Work out the finished part from the listing and answer in its coordinate system (mm). Face numbers are marked on the shaded views. Round coordinates to 2 decimals unless told otherwise and drop trailing zeros. Order: outer loops, then holes, each group sorted by start corner. A loop starts at its lowest first (then second) coordinate and runs counter-clockwise, first axis right, second up. Notation, with made-up numbers: (36, 84.5) -> (47, 84.5) arc R25 cw to (47, 102.5) -> close; hole circle Ø2 at (28, 47). An arc over 180 degrees is marked (long way). Use one line per item in the form item = value.
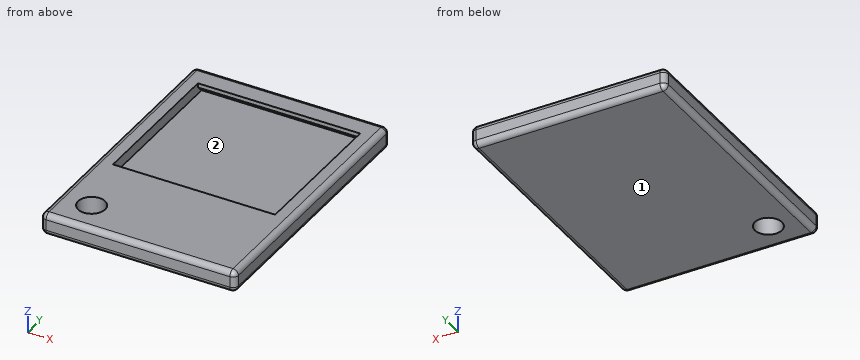
```python
from build123d import *

# Parameters (mm, degrees)
F0_W          = 36
F0_H          = 50
F1_DEPTH      = 4
F2_W          = 30
F2_H          = 30
F3_DEPTH      = 2
F4_R          = 1
F6_DEPTH      = 15
F6_DEPTH_BACK = 15
F8_DEPTH      = 15
F8_DEPTH_BACK = 15
F9_R          = 2.5
F10_DEPTH     = 4.001


with BuildPart() as f1:
    # F0 (on Top) → F1 (new body)
    with BuildSketch(Plane.XY):
        Rectangle(F0_W, F0_H)
    extrude(amount=F1_DEPTH)

    # F2 (on face) → F3 (cut)
    with BuildSketch(Plane.XY.offset(4)):
        with Locations((0, 7)):
            Rectangle(F2_W, F2_H)
    extrude(amount=-F3_DEPTH, mode=Mode.SUBTRACT)

    # F4
    f4_edges = [f1.edges().sort_by_distance(p)[0] for p in [
        (0, -25, 4),
        (18, 0, 4),
        (0, 25, 4),
        (-18, 0, 4),
        (18, -25, 2),
        (-18, -25, 2),
        (18, 25, 2),
        (18, 0, 0),
        (0, -25, 0),
        (-18, 0, 0),
        (0, 25, 0),
        (-18, 25, 2),
    ]]
    fillet(f4_edges, radius=F4_R)

    # F5 (on Right) → F6 (join, two sides)
    with BuildSketch(Plane.YZ) as f6_sk:
        Polygon((-6.8, 4), (-8, 4), (-8, 2), (-6.8, 3.2), align=None)
    extrude(amount=F6_DEPTH)
    extrude(f6_sk.sketch, amount=-F6_DEPTH_BACK)

    # F7 (on Right) → F8 (join, two sides)
    with BuildSketch(Plane.YZ) as f8_sk:
        Polygon((22, 2), (22, 4), (20.8, 4), (20.8, 3.2), align=None)
    extrude(amount=F8_DEPTH)
    extrude(f8_sk.sketch, amount=-F8_DEPTH_BACK)

    # F9 (on face) → F10 (cut, through all)
    with BuildSketch(Plane.XY.offset(4)):
        with Locations((-12, -19)):
            Circle(F9_R)
    extrude(amount=-F10_DEPTH, mode=Mode.SUBTRACT)


solid = f1.part
```
Item 1: The part is cut by section A-A, the plane y = -19. Give the vertices of the cut face in (x, z), and give its area (3 significant figures).
Findings:
outline = (-18, 1) arc R1 ccw to (-17, 0) -> (-14.5, 0) -> (-14.5, 4) -> (-17, 4) arc R1 ccw to (-18, 3) -> close; (-9.5, 0) -> (17, 0) arc R1 ccw to (18, 1) -> (18, 3) arc R1 ccw to (17, 4) -> (-9.5, 4) -> close
area = 123 mm^2
Item 2: Flat-ended cylindrical pins translate along their axes: P1, Ø10, axis at x = 4.5, y = 9.5, coming from the +Z side; P2, Ø0.6, axis at x = -6, z = 3.5, coming from the -Y side; P3, Ø4.5, axis at x = -12, y = -19, coming from the +Z side. Find the tip coordinate at first contact, or state that the pin passes through.
Findings:
P1 = 2
P2 = -24.98
P3 = through
Item 3: Consider line 1 along Y through (x, z) = (-12, 1.9); line 2 along Y through (x, z) = (-12, 2.9); line 3 along X through (y, z) = (-6, 2.35). Determine where each line is inside the solid, lowest interval first.
Findings:
line_1 = -25 to -21.5, -16.5 to 25
line_2 = -25 to -21.5, -16.5 to -7.1, 21.1 to 25
line_3 = -18 to -15, 15 to 18
Item 4: The part is cut by section B-B, the plane x = -13.5. Give the vertices of the cut face in (y, z).
Findings:
outline = (-25, 1) arc R1 ccw to (-24, 0) -> (-21, 0) -> (-21, 4) -> (-24, 4) arc R1 ccw to (-25, 3) -> close; (-17, 0) -> (24, 0) arc R1 ccw to (25, 1) -> (25, 3) arc R1 ccw to (24, 4) -> (20.8, 4) -> (20.8, 3.2) -> (22, 2) -> (-8, 2) -> (-6.8, 3.2) -> (-6.8, 4) -> (-17, 4) -> close
Item 5: Determine the mould class of the marked faces 1 and 2 for opening direction X: released by +X, released by -X, zero draft, split by the parting line, or undercut.
Findings:
face_1 = zero draft
face_2 = undercut
Item 6: The part is cut by section C-C, the plane y = 16. Give the vertices of the cut face in (x, z), and give its area (3 significant figures).
Findings:
outline = (-18, 1) arc R1 ccw to (-17, 0) -> (17, 0) arc R1 ccw to (18, 1) -> (18, 3) arc R1 ccw to (17, 4) -> (15, 4) -> (15, 2) -> (-15, 2) -> (-15, 4) -> (-17, 4) arc R1 ccw to (-18, 3) -> close
area = 83.1 mm^2
Item 7: The part is cut by section D-D, the plane x = -1. Give the vertices of the cut face in (y, z).
Findings:
outline = (-25, 1) arc R1 ccw to (-24, 0) -> (24, 0) arc R1 ccw to (25, 1) -> (25, 3) arc R1 ccw to (24, 4) -> (20.8, 4) -> (20.8, 3.2) -> (22, 2) -> (-8, 2) -> (-6.8, 3.2) -> (-6.8, 4) -> (-24, 4) arc R1 ccw to (-25, 3) -> close
